Autodesk Inventor part; units mm, degrees
ref_plane "作業平面1" through (0, 0, 0) normal (0, 0, -1) x (-1, 0, 0)
ref_plane "YZ Plane" through (0, 0, 0) normal (1, 0, 0) x (0, 1, 0)
ref_plane "XZ Plane" through (0, 0, 0) normal (0, 1, 0) x (-1, 0, 0)
sketch "スケッチ1" plane through (0, 0, 0) normal (0, 0, 1) x (1, 0, 0)
  circle A0 centre (0, 0) radius 5
  circle A1 centre (0, 0) radius 4.5
  dimension "d0" = 10
  dimension "d10" = 9
ref_plane "作業平面1" through (0, 0, 0) normal (0, 0, -1) x (-1, 0, 0)
sketch "スケッチ2" plane through (0, 0, 0) normal (0, 0, -1) x (-1, 0, 0)
  line L0 (-5.5874, 2.4478) -> (5.5874, 2.4478) construction
  line L1 (5.5874, 2.4478) -> (5.5874, -2.4478) construction
  line L2 (5.5874, -2.4478) -> (-5.5874, -2.4478) construction
  line L3 (-5.5874, -2.4478) -> (-5.5874, 2.4478) construction
  line L4 (5.5874, 2.4478) -> (-5.5874, -2.4478) construction
  line L5 (5.5874, -2.4478) -> (-5.5874, 2.4478) construction
  line L6 (-2.6039, 0.0543) -> (-0.5793, 0.0543)
  line L7 (-0.5793, 0.0543) -> (-0.5793, 1.222)
  spline S0 degree 2 poles (-0.5793, 1.222) (-0.9655, 1.5328) (-0.9655, 1.5901) knots 0 0 0 1 1 1
  spline S1 degree 2 poles (-0.9655, 1.5901) (-0.9655, 1.6414) (-0.697, 1.9703) knots 0 0 0 1 1 1
  spline S2 degree 2 poles (-0.697, 1.9703) (-0.5612, 2.1392) (-0.5159, 2.1392) knots 0 0 0 1 1 1
  spline S3 degree 2 poles (-0.5159, 2.1392) (-0.4677, 2.1392) (-0.4677, 2.0759) knots 0 0 0 1 1 1
  line L8 (-0.4677, 2.0759) -> (-0.4677, -1.6263)
  spline S4 degree 2 poles (-0.4677, -1.6263) (-0.4677, -1.8888) (-0.4405, -2.0849) knots 0 0 0 1 1 1
  line L9 (-0.4405, -2.0849) -> (-0.6155, -2.1392)
  spline S5 degree 2 poles (-0.6155, -2.1392) (-0.5793, -1.8677) (-0.5793, -1.6293) knots 0 0 0 1 1 1
  line L10 (-0.5793, -1.6293) -> (-0.5793, -0.4375)
  line L11 (-0.5793, -0.4375) -> (-3.7746, -0.4375)
  spline S6 degree 2 poles (-3.7746, -0.4375) (-4.2151, -0.4375) (-4.4504, -0.4677) knots 0 0 0 1 1 1
  spline S7 degree 2 poles (-4.4504, -0.4677) (-4.4142, -0.0151) (-4.3659, 0.1328) knots 0 0 0 1 1 1
  spline S8 degree 2 poles (-4.3659, 0.1328) (-4.3388, 0.2233) (-4.2935, 0.2233) knots 0 0 0 1 1 1
  spline S9 degree 2 poles (-4.2935, 0.2233) (-4.2151, 0.2233) (-4.1578, 0.0543) knots 0 0 0 1 1 1
  line L12 (-4.1578, 0.0543) -> (-2.7155, 0.0543)
  line L13 (-2.7155, 0.0543) -> (-2.7155, 0.8388)
  spline S10 degree 2 poles (-2.7155, 0.8388) (-3.0927, 1.1284) (-3.0927, 1.1888) knots 0 0 0 1 1 1
  spline S11 degree 2 poles (-3.0927, 1.1888) (-3.0927, 1.2401) (-2.8302, 1.5539) knots 0 0 0 1 1 1
  spline S12 degree 2 poles (-2.8302, 1.5539) (-2.6944, 1.7138) (-2.6522, 1.7138) knots 0 0 0 1 1 1
  spline S13 degree 2 poles (-2.6522, 1.7138) (-2.6039, 1.7138) (-2.6039, 1.6504) knots 0 0 0 1 1 1
  line L14 (-2.6039, 1.6504) -> (-2.6039, 0.0543)
  line L15 (4.1034, -1.4) -> (4.2905, -1.4)
  spline S14 degree 2 poles (4.2905, -1.4) (4.4836, -1.4) (4.4836, -1.6866) knots 0 0 0 1 1 1
  spline S15 degree 2 poles (4.4836, -1.6866) (4.4836, -1.8797) (4.3237, -1.8797) knots 0 0 0 1 1 1
  spline S16 degree 2 poles (4.3237, -1.8797) (3.4487, -1.8526) (1.9763, -1.8526) knots 0 0 0 1 1 1
  spline S17 degree 2 poles (1.9763, -1.8526) (1.0651, -1.8526) (0.4164, -1.8767) knots 0 0 0 1 1 1
  spline S18 degree 2 poles (0.4164, -1.8767) (0.5341, -1.5961) (0.6879, -1.3276) knots 0 0 0 1 1 1
  line L16 (0.6879, -1.3276) -> (0.6879, 1.3185)
  spline S19 degree 2 poles (0.6879, 1.3185) (0.4466, 1.5358) (0.4466, 1.5901) knots 0 0 0 1 1 1
  spline S20 degree 2 poles (0.4466, 1.5901) (0.4466, 1.6414) (0.6397, 1.8677) knots 0 0 0 1 1 1
  spline S21 degree 2 poles (0.6397, 1.8677) (0.7392, 1.9823) (0.7875, 1.9823) knots 0 0 0 1 1 1
  spline S22 degree 2 poles (0.7875, 1.9823) (0.8478, 1.9823) (0.9444, 1.8405) knots 0 0 0 1 1 1
  line L17 (0.9444, 1.8405) -> (1.4935, 1.8405)
  spline S23 degree 2 poles (1.4935, 1.8405) (2.9237, 1.8405) (4.2573, 1.8737) knots 0 0 0 1 1 1
  spline S24 degree 2 poles (4.2573, 1.8737) (4.4685, 1.8737) (4.4685, 1.575) knots 0 0 0 1 1 1
  spline S25 degree 2 poles (4.4685, 1.575) (4.4685, 1.3728) (4.3056, 1.3728) knots 0 0 0 1 1 1
  line L18 (4.3056, 1.3728) -> (4.1034, 1.3728)
  line L19 (4.1034, 1.3728) -> (4.1034, -1.4)
  line L20 (3.9948, 1.3728) -> (2.3776, 1.3728)
  line L21 (2.3776, 1.3728) -> (2.3776, 0.1901)
  line L22 (2.3776, 0.1901) -> (3.9948, 0.1901)
  line L23 (3.9948, 0.1901) -> (3.9948, 1.3728)
  line L24 (2.3776, -1.4) -> (3.9948, -1.4)
  line L25 (3.9948, -1.4) -> (3.9948, -0.2685)
  line L26 (3.9948, -0.2685) -> (2.3776, -0.2685)
  line L27 (2.3776, -0.2685) -> (2.3776, -1.4)
  line L28 (2.269, 1.3728) -> (0.7996, 1.3728)
  line L29 (0.7996, 1.3728) -> (0.7996, 0.1901)
  line L30 (0.7996, 0.1901) -> (2.269, 0.1901)
  line L31 (2.269, 0.1901) -> (2.269, 1.3728)
  line L32 (2.269, -1.4) -> (2.269, -0.2685)
  line L33 (2.269, -0.2685) -> (0.7996, -0.2685)
  line L34 (0.7996, -0.2685) -> (0.7996, -1.4)
  line L35 (0.7996, -1.4) -> (2.269, -1.4)
  point P0 (0, 0)
  point P1 (0, 0)
extrude "押し出し5" add sketch "スケッチ1" against normal blind 1
sketch "スケッチ3" plane through (0, 0, -1) normal (0, 0, -1) x (-1, 0, 0)
  circle A0 centre (0, 0) radius 5
extrude "押し出し6" add sketch "スケッチ3" along normal blind 59
fillet "フィレット2" radius 1 1 edges at (5, 0, -60)
extrude "押し出し9" add sketch "スケッチ2" along normal blind 1
properties part number "ueda_hanko"
The listing builds one solid part. Answer for the finished solid, in the listing's coordinates (mm). Coordinates: 2 decimals unless noted, no trailing zeros. Write each loop counter-clockwise with the first axis right and the second up, starting at its lowest first coordinate (ties: lowest second). Pieces come first, ordered by that corner, then holes. Notation, with made-up numbers: (45.25, 54.5) - (60.25, 54.5) arc R11 ccw to (60.25, 70.5) - close; hole circle Ø3 at (-19, 64). An arc over 180 degrees is marked (long way). One line per item, written item: value.
1) Each of these flat-tipped pins is pushed along its axis until it touches: pin 1 Ø0.5 at (y, z) = (1, -0.5) entering from -X; pin 2 Ø1.1 at (y, z) = (1, -0.5) entering from -X; pin 3 Ø3 at (x, z) = (2.5, -47.5) entering from +Y; pin 4 Ø0.8 at (y, z) = (0.5, -0.5) entering from +X. Where does it stop, or does it pass through?
Geometry check:
pin 1: stops at x = -4.94
pin 2: stops at x = -4.98
pin 3: stops at y = 4.9
pin 4: stops at x = 5
2) For a pull along X with two mould halves and no side action, classify faces 1 (the flat face through (-1, 0, 0)), 2 (the flat face through (-2, -1, -1)), 3 (the flat face through (-3.2, 0.19, -0.5)) as pulls with the +X half, pulls with the -X half, needs draft (parallel to the pull), parting line crosses it, or undercut.
Geometry check:
face 1: needs draft
face 2: undercut
face 3: undercut
3) Find section A-A (z = -39.5). Give the vertices of the cut face in (x, y).
Geometry check:
outline: circle Ø10 at (0, 0)
4) Consider line 1 along Y through (x, z) = (-3, -42.5); line 2 along X through (y, z) = (-0.25, -9); line 3 along Y through (x, z) = (0, -0.55). Determine where each line is inside the solid, lowest interval first. Write a range as from..to.
Geometry check:
line 1: y = -4..4
line 2: x = -4.99..4.99
line 3: y = -5..-4.5, 4.5..5
